Drawing for the job (mm, zero at the part's lowest x, y, z). Coordinates: 2 decimals unless noted, no trailing zeros. Write each loop counter-clockwise with the first axis right and the second up, starting at its lowest first coordinate (ties: lowest second). Pieces come first, ordered by that corner, then holes. Notation, with made-up numbers: (36.25, 37) -> (49.25, 37) arc R18 cw to (49.25, 71) -> close; hole circle Ø3 at (57.25, 36). An arc over 180 degrees is marked (long way). Write item = value, one per line. Start each with the question number.
Q1. Band-saw the part on C-C, the plane x = 284. List the corners of the cut face in (y, z).
Q2. Pin check, flat tips, straight feed: P1, Ø1, axis at x = 223, z = 1.5, coming from the -Y side; P2, Ø4, axis at y = 16.5, z = 6, coming from the -X side; P3, Ø6, axis at x = 232.5, y = 18.5, coming from the +Z side. Stop position of each tip, or through.
Q3. Probe line 1 (X direction, y = 20.5, z = 7); line 2 (X direction, y = 18.5, z = 3.5) (1 decimal); line 3 (Y direction, x = 190, z = 7.75). List the from-to ranges inside material, lowest first.
Q4. Band-saw the part on B-B, the plane y = 18. List the corners of the cut face in (x, z), plus the area to 3 significant figures.
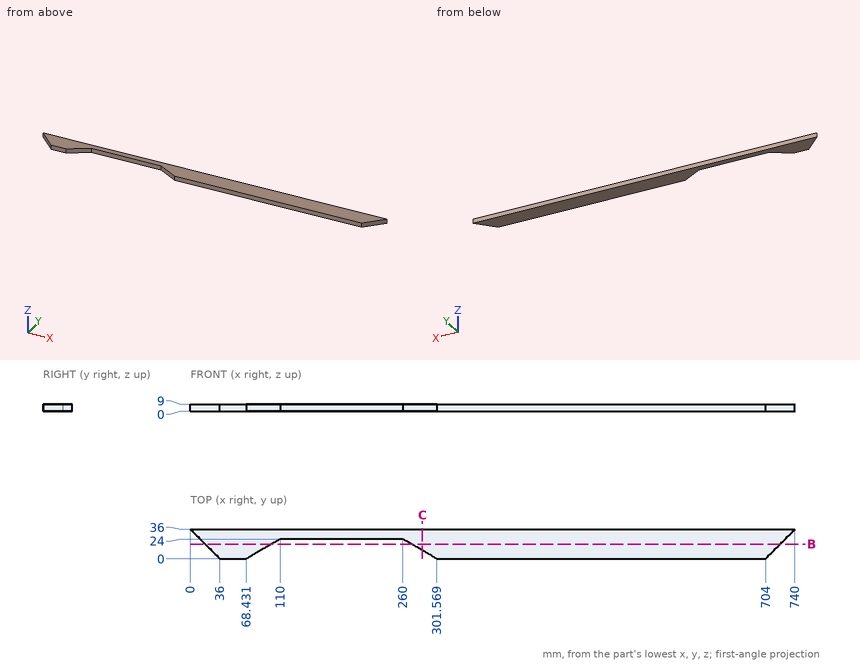
Ans:
q1.outline = (10.14, 0) -> (36, 0) -> (36, 9) -> (10.14, 9) -> close
q2.P1 = 24
q2.P2 = 17.5
q2.P3 = through
q3.line_1 = 15.5 to 103.94, 266.06 to 724.5
q3.line_2 = 17.5 to 100.5, 269.5 to 722.5
q3.line_3 = 24 to 36
q4.outline = (18, 0) -> (99.61, 0) -> (99.61, 9) -> (18, 9) -> close; (270.39, 0) -> (722, 0) -> (722, 9) -> (270.39, 9) -> close
q4.area = 4,800 mm2
